from build123d import *

# Parameters (mm, degrees)
F1_DEPTH = 14
F2_R     = 6.99999
F3_R     = 3
F4_DEPTH = 25
F5_R     = 3
F6_DEPTH = 25


# Not quite as in the source:
# - a fillet or chamfer is up to 0.001 mm smaller than in the source, because OpenCascade refuses the exact size


with BuildPart() as f1:
    # F0 (on Front) → F1 (new body)
    with BuildSketch(Plane.XZ):
        with BuildLine():
            Line((3, 0), (41, 0))
            Line((41, 0), (41, 1.5))
            Line((41, 1.5), (3, 1.5))
            ThreePointArc((3, 1.5), (1.9393398282, 1.9393398282), (1.5, 3))
            Line((1.5, 3), (1.5, 41))
            Line((1.5, 41), (0, 41))
            Line((0, 41), (0, 3))
            ThreePointArc((0, 3), (0.8786796564, 0.8786796564), (3, 0))
        make_face()
    extrude(amount=F1_DEPTH)

    # F2 (radius 7 in the source; OpenCascade refuses exactly that, so slightly less here)
    f2_edges = [f1.edges().sort_by_distance(p)[0] for p in [
        (41, 0, 0.75),
        (41, -14, 0.75),
        (0.75, 0, 41),
        (0.75, -14, 41),
    ]]
    fillet(f2_edges, radius=F2_R)

    # F3 (on face) → F4 (cut)
    with BuildSketch(Plane(origin=(0, 0, 0), x_dir=(0, -1, 0), z_dir=(-1, 0, 0))):
        with Locations((7, 15)):
            Circle(F3_R)
        with Locations((7, 35)):
            Circle(F3_R)
    extrude(amount=-F4_DEPTH, mode=Mode.SUBTRACT)

    # F5 (on face) → F6 (cut)
    with BuildSketch(Plane(origin=(0, 0, 0), x_dir=(1, 0, 0), z_dir=(0, 0, -1))):
        with Locations((35, 7)):
            Circle(F5_R)
        with Locations((15, 7)):
            Circle(F5_R)
    extrude(amount=-F6_DEPTH, mode=Mode.SUBTRACT)


solid = f1.part
Work out the finished part from the listing and answer in its coordinate system (mm). A direction names the side the tool comes from. Round coordinates to 2 decimals unless told otherwise and drop trailing zeros. Write each loop counter-clockwise with the first axis right and the second up, starting at its lowest first coordinate (ties: lowest second). Pieces come first, ordered by that corner, then holes.
1) A cutting plane is placed at D-D (z = 29). Give the vertices of the cut face in (x, y).
2) A tool of negligible diameter and unlimited length cuts with its end or side. For faces 1 (the flat face through (22, -7, 1.5)), 2 (the flat face through (0, -7, 22)), from which of +Z, -Z, +X, -X, +Y, -Y can it reach the whole face along a straight path? Write none if from no direction.
3) A cutting plane is placed at B-B (x = 14.5). Give the vertices of the cut face in (y, z), plus the area to 3 significant figures.
4) Straight lines are drawn through the part: line 1 (Y direction, x = 15, z = 0.3); line 2 (Z direction, x = 1.25, y = -7); line 3 (Z direction, x = 1, y = -7). For each, find the intervals that lie inside material, in ascending order.
5) A cutting plane is placed at A-A (z = 15). Give the vertices of the cut face in (x, y).
6) A cutting plane is placed at C-C (y = -8.5). Give the vertices of the cut face in (x, z).
7) The mould has two halves that part along Z. Classify faces 3 (the cylindrical face through (0.74, -8.61, 37.53)), 4 (the flat face through (9, 0, 1)), 5 (the cylindrical face through (0.7, -2.1, 39)), 6 (the cylindrical face through (0.74, -8.384, 12.338)): pulls with the +Z half, pulls with the -Z half, needs draft (parallel to the pull), parting line crosses it, or undercut.
8) Given pin 1 Ø6 at (x, y) = (30, -8) entering from +Z; pin 2 Ø5.5 at (x, y) = (35, -7) entering from -Z; pin 3 Ø7 at (y, z) = (-10, 23.5) entering from +X, each flat-ended and moving along its own axis, determine where each tip first touches the part or whether it passes through.
Completed:
1. outline: (0, -14) - (1.5, -14) - (1.5, 0) - (0, 0) - close
2. face 1: +Z, +X, +Y, -Y
2. face 2: +Z, -Z, -X, +Y, -Y
3. outline: (-14, 0) - (-9.96, 0) - (-9.96, 1.5) - (-14, 1.5) - close; (-4.04, 0) - (0, 0) - (0, 1.5) - (-4.04, 1.5) - close
3. area: 12.1 mm2
4. line 1: y = -14 to -10, -4 to 0
4. line 2: z = 0.56 to 12, 18 to 32, 38 to 41
4. line 3: z = 0.76 to 12, 18 to 32, 38 to 41
5. outline: (0, -14) - (1.5, -14) - (1.5, -10) - (0, -10) - close; (0, -4) - (1.5, -4) - (1.5, 0) - (0, 0) - close
6. outline: (0, 3) arc R3 ccw to (3, 0) - (12.4, 0) - (12.4, 1.5) - (3, 1.5) arc R1.5 cw to (1.5, 3) - (1.5, 12.4) - (0, 12.4) - close; (0, 17.6) - (1.5, 17.6) - (1.5, 32.4) - (0, 32.4) - close; (0, 37.6) - (1.5, 37.6) - (1.5, 40.84) - (0, 40.84) - close; (17.6, 0) - (32.4, 0) - (32.4, 1.5) - (17.6, 1.5) - close; (37.6, 0) - (40.84, 0) - (40.84, 1.5) - (37.6, 1.5) - close
7. face 3: undercut
7. face 4: needs draft
7. face 5: pulls with the +Z half
7. face 6: undercut
8. pin 1: stops at z = 1.5
8. pin 2: passes through
8. pin 3: stops at x = 1.5
